Can you work these out from the model? Positions are in its coordinate system, mm. A direction names the side the tool comes from. Round coordinates to 2 decimals unless told otherwise and drop trailing zeros. Loops run counter-clockwise (first coordinate to the right, second up) from the corner with the lowest first, then second, coordinate; pieces in that order, holes last. Notation, with made-up numbers: (-17.75, 31) -> (-10.75, 31) arc R30 ccw to (-10.75, 68) -> close; hole circle Ø5 at (70, -21). An arc over 180 degrees is marked (long way). Answer as a JSON object with one key per item and string values.
```python
from build123d import *

# Parameters (mm, degrees)
SKETCH1_R           = 3.175
BOSS_EXTRUDE1_DEPTH = 25.4
FILLET1_R           = 6.35
CUT_EXTRUDE1_REACH  = 97.723
SKETCH2_R           = 2.54
CUT_EXTRUDE2_REACH  = 69.917
SKETCH3_R           = 1.5875
FILLET2_R           = 2.54


with BuildPart() as part:
    # Sketch1 → Boss-Extrude1 (new body)
    with BuildSketch(Plane(origin=(0, 0, 0), x_dir=(0, 0, -1), z_dir=(1, 0, 0))):
        with BuildLine():
            Line((-9.510223779, 67.442100456), (18.518782335, 87.194732923))
            Line((18.518782335, 87.194732923), (24.971703957, 87.705940953))
            Line((24.971703957, 87.705940953), (25.834610798, 76.813564689))
            Line((25.834610798, 76.813564689), (1.957775741, 59.987054843))
            Line((1.957775741, 59.987054843), (-4.791410802, 25.984772629))
            Line((-4.791410802, 25.984772629), (3.587814077, 7.472662593))
            Line((3.587814077, 7.472662593), (19.957119618, 11.661325034))
            ThreePointArc((19.957119618, 11.661325034), (27.683063897, 7.083685359), (23.105424222, -0.64225892))
            Line((23.105424222, -0.64225892), (-3.587814077, -7.472662593))
            Line((-3.587814077, -7.472662593), (-18.041777156, 24.460285718))
            Line((-18.041777156, 24.460285718), (-9.510223779, 67.442100456))
        make_face()
        Circle(SKETCH1_R, mode=Mode.SUBTRACT)
    extrude(amount=BOSS_EXTRUDE1_DEPTH)

    # Fillet1
    fillet1_edges = [part.edges().sort_by_distance(p)[0] for p in [
        (12.7, 67.442100456, 9.510223779),
        (12.7, 87.194732923, -18.518782335),
        (12.7, 59.987054843, -1.957775741),
        (12.7, 25.984772629, 4.791410802),
        (12.7, 7.472662593, -3.587814077),
        (12.7, -7.472662593, 3.587814077),
        (12.7, 24.460285718, 18.041777156),
    ]]
    fillet(fillet1_edges, radius=FILLET1_R)

    # Sketch2 → Cut-Extrude1 (cut, up to next)
    with BuildSketch(Plane(origin=(0, -6.151791977, -1.574152302), x_dir=(1, 0, 0), z_dir=(0, -0.968786138, -0.247898)), mode=Mode.PRIVATE) as cut_extrude1_sk1:
        with Locations((12.7, -18.415)):
            Circle(SKETCH2_R)
    cut_extrude1_tool1 = extrude(cut_extrude1_sk1.sketch, amount=-CUT_EXTRUDE1_REACH, mode=Mode.PRIVATE) & part.part
    add(cut_extrude1_tool1.solids().sort_by_distance((12.7, -1.58675, -19.414349))[0], mode=Mode.SUBTRACT)

    # Sketch3 → Cut-Extrude2 (cut, up to next)
    with BuildSketch(Plane(origin=(0, -2.618484858, 5.784983755), x_dir=(1, 0, 0), z_dir=(0, -0.41235982, 0.911021064)), mode=Mode.PRIVATE) as cut_extrude2_sk1:
        with Locations((12.7, 21.336)):
            Circle(SKETCH3_R)
    cut_extrude2_tool1 = extrude(cut_extrude2_sk1.sketch, amount=-CUT_EXTRUDE2_REACH, mode=Mode.PRIVATE) & part.part
    add(cut_extrude2_tool1.solids().sort_by_distance((12.7, 16.819061, 14.583093))[0], mode=Mode.SUBTRACT)

    # Fillet2
    fillet2_edges = [part.edges().sort_by_distance(p)[0] for p in [
        (12.7, 87.705940953, -24.971703957),
        (12.7, 76.813564689, -25.834610798),
    ]]
    fillet(fillet2_edges, radius=FILLET2_R)


solid = part.part
```
Q1. I want a section at C-C, the plane z = -12.5. Write out the boundary of the cut face in (x, y), then the cut area to 3 significant figures.
Determined:
{"outline": "(0, -3.36) -> (25.4, -3.36) -> (25.4, 9.75) -> (0, 9.75) -> close; (0, 67.42) -> (25.4, 67.42) -> (25.4, 82.95) -> (0, 82.95) -> close", "area": "728 mm²"}
Q2. I'm going to push flat-ended pins straight in: pin 1 (5 mm diameter, centred on x = 5.5, y = 17, fed in from -Z); pin 2 (10 mm diameter, centred on y = 20, z = -2.5, fed in from -X); pin 3 (8 mm diameter, centred on x = 18.5, z = -6.5, fed in from -Y); pin 4 (1.5 mm diameter, centred on x = 4, y = 68, fed in from -Z). Where does each tip first touch, or does it pass through?
Determined:
{"pin 1": "z = -0.41", "pin 2": "x = 0", "pin 3": "y = -5.91", "pin 4": "z = -14.39"}
Q3. On a 3-axis mill with a long thin cutter (end or side, diameter ignored), from which of +Z, -Z, +X, -X, +Y, -Y can I reach the whole of each face in a straight line? I mean faces 5 (the flat face through (12.52, -3.36, -12.49)), 6 (the cylindrical face through (12.878, 9.194, -4.483)), 7 (the flat face through (12.522, 42.946, 1.425)). Say none if no direction works.
Determined:
{"face 5": "-Z, +X, -X, -Y", "face 6": "+X, -X", "face 7": "-Z, +X, -X"}
Q4. I want a section at B-B, the plane z = 0. Write out the boundary of the cut face in (x, y) (3 decimals).
Determined:
{"outline": "(0, -6.35) -> (25.4, -6.35) -> (25.4, -3.175) -> (0, -3.175) -> close; (0, 3.175) -> (25.4, 3.175) -> (25.4, 15.399) -> (0, 15.399) -> close; (0, 50.124) -> (25.4, 50.124) -> (25.4, 74.144) -> (0, 74.144) -> close"}
Q5. We'd pull the mould along Y, two halves only. Please class faces 1 (the cylindrical face through (12.88, 86.92, -24.27)), 2 (the flat face through (12.522, 9.816, 11.413)), 3 (the cylindrical face through (10.684, 4.862, -19.36)), 4 (the flat face through (0, 31, 5)): pulls with the +Y half, pulls with the -Y half, needs draft (parallel to the pull), parting line crosses it, or undercut.
Determined:
{"face 1": "pulls with the +Y half", "face 2": "pulls with the -Y half", "face 3": "undercut", "face 4": "needs draft"}
Q6. If I drill on L1, parallel to Y at x = 7, z = -2; L2, parallel to Y at x = 9, z = -10; L3, parallel to X at y = 18, z = 11, over which ranges is the centre line in solid material (lowest first)? Write a range as [from, to].
Determined:
{"L1": "[-6.04, -2.47], [2.47, 11.27], [59.07, 75.55]", "L2": "[-4, 9.11], [65.65, 81.19]", "L3": "[0, 11.16], [14.24, 25.4]"}
Q7. I want a section at D-D, the plane y = 74. Write out the boundary of the cut face in (x, z), then the cut area to 3 significant figures.
Determined:
{"outline": "(0, -21.84) -> (25.4, -21.84) -> (25.4, 0.2) -> (0, 0.2) -> close", "area": "560 mm²"}
Q8. I want a section at A-A, the plane x = 6. Write out the boundary of the cut face in (y, z) (3 decimals).
Determined:
{"outline": "(-6.152, -1.574) -> (-0.642, -23.105) arc R6.35 ccw to (11.661, -19.957) -> (8.794, -8.75) arc R6.35 cw to (12.327, -1.391) -> (24.129, 3.951) arc R6.35 cw to (27.983, 4.395) -> (57.496, -1.463) arc R6.35 cw to (61.45, -4.034) -> (75.98, -24.651) arc R2.54 ccw to (78.257, -25.72) -> (85.174, -25.172) arc R2.54 ccw to (87.505, -22.44) -> (87.332, -20.253) arc R6.35 ccw to (86.193, -17.097) -> (68.905, 7.434) arc R6.35 ccw to (64.951, 10.005) -> (26.459, 17.645) arc R6.35 ccw to (22.604, 17.202) -> (-2.618, 5.785) arc R6.35 ccw to start; hole circle Ø6.35 at (0, 0)"}
